```python
from build123d import *
from OCP.BRepFilletAPI import BRepFilletAPI_MakeChamfer

# Parameters (mm, degrees)
BOSS_EXTRU_1_DEPTH      = 200
BOSS_EXTRU_2_DEPTH      = 50
BOSS_EXTRU_2_DEPTH_BACK = 90
ESQUISSE3_W             = 40
ESQUISSE3_H             = 110
BOSS_EXTRU_3_DEPTH      = 150
CHANFREIN1_SIZE         = 10
CHANFREIN1_SIZE2        = 17.320508076
CHANFREIN2_SIZE         = 100
CHANFREIN2_SIZE2        = 46.630765816
CHANFREIN3_SIZE         = 10
CHANFREIN4_SIZE         = 30
BOSS_EXTRU_4_DEPTH      = 10
ENL_V_MAT_EXTRU_1_DEPTH = 130
ESQUISSE7_R             = 10
BOSS_EXTRU_5_DEPTH      = 30
CHANFREIN5_SIZE         = 27.474774195
CHANFREIN5_SIZE_2       = 10
ENL_V_MAT_EXTRU_2_DEPTH = 130
CHANFREIN6_SIZE         = 10
CHANFREIN6_SIZE_2       = 27.474774195
CHANFREIN6_SIZE_3       = 9.402654051


# Some blends are built 0.0001 mm under size
with BuildPart() as part:
    # Esquisse1 → Boss.-Extru.1 (new body)
    with BuildSketch(Plane.XY):
        Polygon((-42.05848897, 40), (-42.05848897, 0), (-37.05848897, 0), (-37.05848897, 5), (-37.05848897, 39.208077798), (-29.772778292, 61.631189606), (-11.372189368, 75), (11.372189368, 75), (29.772778292, 61.631189606), (37.05848897, 39.208077798), (37.05848897, 5), (37.05848897, 0), (42.05848897, 0), (42.05848897, 40), (34.026032334, 64.72135955), (12.996787849, 80), (-12.996787849, 80), (-34.026032334, 64.72135955), align=None)
    extrude(amount=BOSS_EXTRU_1_DEPTH)

    # Esquisse3 → Boss.-Extru.2 (add, two sides: drawn at the far end of the back side and taken through both)
    with BuildSketch(Plane(origin=(42.05848897, 0, 0), x_dir=(0, 0, -1), z_dir=(1, 0, 0)).offset(-BOSS_EXTRU_2_DEPTH_BACK)):
        with Locations((20, 45)):
            Rectangle(ESQUISSE3_W, ESQUISSE3_H)
    extrude(amount=BOSS_EXTRU_2_DEPTH + BOSS_EXTRU_2_DEPTH_BACK)

    # Esquisse4 → Boss.-Extru.3 (add)
    with BuildSketch(Plane.XY):
        Polygon((42.05848897, 40), (42.05848897, 15), (82.05848897, 15), (82.05848897, 65), (33.642516656, 65), (34.026032334, 64.72135955), align=None)
    extrude(amount=BOSS_EXTRU_3_DEPTH)

    # Chanfrein1: one chamfer whose edges measure the first distance from different faces: ONE call of the kernel's chamfer builder (chamfer() names one face for all edges)
    chanfrein1_edges_1 = [part.edges().sort_by_distance(p)[0] for p in [
        (92.05848897, -10, -20),
    ]]
    chanfrein1_side_1 = [part.faces().sort_by_distance(p)[0] for p in [
        (22.05848897, -10, -20),
    ]]
    chanfrein1_edges_2 = [part.edges().sort_by_distance(p)[0] for p in [
        (92.05848897, 100, -20),
    ]]
    chanfrein1_side_2 = [part.faces().sort_by_distance(p)[0] for p in [
        (22.05848897, 100, -20),
    ]]
    chanfrein1 = BRepFilletAPI_MakeChamfer(part.part.solid().wrapped)
    for e in chanfrein1_edges_1:
        chanfrein1.Add(CHANFREIN1_SIZE, CHANFREIN1_SIZE2, e.wrapped, chanfrein1_side_1[0].wrapped)  # the first distance lies on this face
    for e in chanfrein1_edges_2:
        chanfrein1.Add(CHANFREIN1_SIZE, CHANFREIN1_SIZE2, e.wrapped, chanfrein1_side_2[0].wrapped)  # the first distance lies on this face
    add(Compound.cast(chanfrein1.Shape()), mode=Mode.REPLACE)

    # Chanfrein2
    chanfrein2_edges = [part.edges().sort_by_distance(p)[0] for p in [
        (82.05848897, 40, 150),
    ]]
    chanfrein2_side = [part.faces().sort_by_distance(p)[0] for p in [
        (82.05848897, 40, 75),
    ]]
    chamfer(chanfrein2_edges, length=CHANFREIN2_SIZE, length2=CHANFREIN2_SIZE2, reference=chanfrein2_side[0])

    # Chanfrein3
    # the kernel refuses this chamfer: 10 mm, written as the material it takes off along each edge
    with BuildSketch(Plane(origin=(92.926890911, 15, 26.692636822), x_dir=(0.02491972708357348, 0.9996219169112968, 0.011620259578202877), z_dir=(-0.4226182617407005, 0, 0.9063077870366495))) as chanfrein3_piece_1_section:
        Polygon((CHANFREIN3_SIZE * 0.999621916911, CHANFREIN3_SIZE * 0.0274958766106), (-CHANFREIN3_SIZE * 0.0274958766106, CHANFREIN3_SIZE * 0.999621916911), (0, 0), align=None)
    chanfrein3_piece_1 = extrude(amount=146.081723085, mode=Mode.PRIVATE)
    chanfrein3_piece_1 = split(chanfrein3_piece_1, bisect_by=Plane(origin=(42.05848897, 18.333333333, 85.0027998), z_dir=(1, 0, 0)), keep=Keep.TOP, mode=Mode.PRIVATE)
    add(chanfrein3_piece_1, mode=Mode.SUBTRACT)
    with BuildSketch(Plane(origin=(82.05848897, 15, 0), x_dir=(0.027495876610586334, 0.9996219169112968, 0), z_dir=(0, 0, 1)), Plane(origin=(82.05848897, 65, 0), x_dir=(-0.9996219169112968, 0.027495876610586317, 0), z_dir=(0, 0, 1))) as chanfrein3_piece_2:
        Polygon((CHANFREIN3_SIZE * 0.999621916911, CHANFREIN3_SIZE * 0.0274958766106), (-CHANFREIN3_SIZE * 0.0274958766106, CHANFREIN3_SIZE * 0.999621916911), (0, 0), align=None)
    extrude(amount=75.71682988, mode=Mode.SUBTRACT)
    with BuildSketch(Plane(origin=(61.144553034, 65, 150), x_dir=(0, 0.027495876610586282, -0.9996219169112968), z_dir=(-1, 0, 0))) as chanfrein3_piece_3_section:
        Polygon((CHANFREIN3_SIZE * 0.999621916911, CHANFREIN3_SIZE * 0.0274958766106), (-CHANFREIN3_SIZE * 0.0274958766106, CHANFREIN3_SIZE * 0.999621916911), (0, 0), align=None)
    chanfrein3_piece_3 = extrude(amount=53.218866257, mode=Mode.PRIVATE)
    chanfrein3_piece_3 = split(chanfrein3_piece_3, bisect_by=Plane(origin=(34.447587874, 63.423945004, 144.130905286), z_dir=(0.9510565162951539, 0.3090169943749468, 0)), keep=Keep.TOP, mode=Mode.PRIVATE)
    add(chanfrein3_piece_3, mode=Mode.SUBTRACT)
    with BuildSketch(Plane(origin=(61.144553034, 65, 150), x_dir=(0, 0.027495876610586282, -0.9996219169112968), z_dir=(-1, 0, 0))) as chanfrein3_piece_4_section:
        Polygon((CHANFREIN3_SIZE * 0.999621916911, CHANFREIN3_SIZE * 0.0274958766106), (-CHANFREIN3_SIZE * 0.0274958766106, CHANFREIN3_SIZE * 0.999621916911), (0, 0), align=None)
    chanfrein3_piece_4 = extrude(amount=53.218866257, mode=Mode.PRIVATE)
    chanfrein3_piece_4 = split(chanfrein3_piece_4, bisect_by=Plane(origin=(33.833825058, 64.86100631, 145.046222385), z_dir=(0.5877852522924745, 0.8090169943749465, 0)), keep=Keep.TOP, mode=Mode.PRIVATE)
    add(chanfrein3_piece_4, mode=Mode.SUBTRACT)
    with BuildSketch(Plane(origin=(92.926890911, 65, 26.692636822), x_dir=(-0.9059651273892109, 0.027495876610586337, -0.4224584769229591), z_dir=(-0.4226182617407005, 0, 0.9063077870366495))) as chanfrein3_piece_5_section:
        Polygon((CHANFREIN3_SIZE * 0.999621916911, CHANFREIN3_SIZE * 0.0274958766106), (-CHANFREIN3_SIZE * 0.0274958766106, CHANFREIN3_SIZE * 0.999621916911), (0, 0), align=None)
    chanfrein3_piece_5 = extrude(amount=161.771451656, mode=Mode.PRIVATE)
    chanfrein3_piece_5 = split(chanfrein3_piece_5, bisect_by=Plane(origin=(37.356602315, 54.470919151, 89.132837903), z_dir=(0.9510565162951539, 0.3090169943749468, 0)), keep=Keep.TOP, mode=Mode.PRIVATE)
    add(chanfrein3_piece_5, mode=Mode.SUBTRACT)
    with BuildSketch(Plane(origin=(92.926890911, 65, 26.692636822), x_dir=(-0.9059651273892109, 0.027495876610586337, -0.4224584769229591), z_dir=(-0.4226182617407005, 0, 0.9063077870366495))) as chanfrein3_piece_6_section:
        Polygon((CHANFREIN3_SIZE * 0.999621916911, CHANFREIN3_SIZE * 0.0274958766106), (-CHANFREIN3_SIZE * 0.0274958766106, CHANFREIN3_SIZE * 0.999621916911), (0, 0), align=None)
    chanfrein3_piece_6 = extrude(amount=161.771451656, mode=Mode.PRIVATE)
    chanfrein3_piece_6 = split(chanfrein3_piece_6, bisect_by=Plane(origin=(33.834404205, 64.860585536, 139.950840197), z_dir=(0.5877852522924745, 0.8090169943749465, 0)), keep=Keep.TOP, mode=Mode.PRIVATE)
    add(chanfrein3_piece_6, mode=Mode.SUBTRACT)

    # Chanfrein4
    chanfrein4_edges = [part.edges().sort_by_distance(p)[0] for p in [
        (-39.55848897, 0, 200),
        (39.55848897, 0, 200),
    ]]
    chamfer(chanfrein4_edges, length=CHANFREIN4_SIZE)

    # Esquisse6 → Boss.-Extru.4 (add)
    with BuildSketch(Plane.XY):
        Polygon((-47.94151103, -10), (82.05848897, -10), (92.05848897, 7.320508076), (92.05848897, 82.679491924), (82.05848897, 100), (-47.94151103, 100), align=None)
    extrude(amount=BOSS_EXTRU_4_DEPTH)

    # Esquisse5 → Enlèv. mat.-Extru.1 (cut)
    with BuildSketch(Plane(origin=(0, 100, 0), x_dir=(1, 0, 0), z_dir=(0, 1, 0))):
        Polygon((77.05848897, -10), (77.05848897, 40), (-47.94151103, 40), (-47.94151103, -10), (33.642516656, -10), (67.05848897, -10), align=None)
        Polygon((67.05848897, -43.145928791), (67.05848897, -10), (33.642516656, -10), (33.642516656, -101.029300724), (42.077832628, -96.717119194), align=None)
    extrude(amount=-ENL_V_MAT_EXTRU_1_DEPTH, mode=Mode.SUBTRACT)

    # Esquisse7 → Boss.-Extru.5 (add)
    with BuildSketch(Plane.ZY.offset(-77.05848897)):
        with Locations(Location((-15, 80, 0), (0, 0, 270))):
            Circle(ESQUISSE7_R)
    extrude(amount=BOSS_EXTRU_5_DEPTH)

    # Chanfrein5
    chanfrein5_edges_1 = [part.edges().sort_by_distance(p)[0] for p in [
        (79.55848897, 22.5, 10),
    ]]
    chanfrein5_side_1 = [part.faces().sort_by_distance(p)[0] for p in [
        (79.55848897, 22.5, 10.2),
    ]]
    chanfrein5_edges_2 = [part.edges().sort_by_distance(p)[0] for p in [
        (82.05848897, 40, 10),
    ]]
    chanfrein5_side_2 = [part.faces().sort_by_distance(p)[0] for p in [
        (82.05848897, 40, 10.2),
    ]]
    chanfrein5_edges_3 = [part.edges().sort_by_distance(p)[0] for p in [
        (79.55848897, 57.5, 10),
    ]]
    chanfrein5_side_3 = [part.faces().sort_by_distance(p)[0] for p in [
        (79.55848897, 57.5, 10.2),
    ]]
    chanfrein5_edges_4 = [part.edges().sort_by_distance(p)[0] for p in [
        (67.05848897, 40, 10),
    ]]
    chanfrein5_side_4 = [part.faces().sort_by_distance(p)[0] for p in [
        (67.25848897, 40, 10),
    ]]
    chanfrein5 = BRepFilletAPI_MakeChamfer(part.part.solid().wrapped)
    for e in chanfrein5_edges_1:
        chanfrein5.Add(CHANFREIN5_SIZE - 0.0001, CHANFREIN5_SIZE_2 - 0.0001, e.wrapped, chanfrein5_side_1[0].wrapped)
    for e in chanfrein5_edges_2:
        chanfrein5.Add(CHANFREIN5_SIZE - 0.0001, CHANFREIN5_SIZE_2 - 0.0001, e.wrapped, chanfrein5_side_2[0].wrapped)
    for e in chanfrein5_edges_3:
        chanfrein5.Add(CHANFREIN5_SIZE - 0.0001, CHANFREIN5_SIZE_2 - 0.0001, e.wrapped, chanfrein5_side_3[0].wrapped)
    for e in chanfrein5_edges_4:
        chanfrein5.Add(CHANFREIN5_SIZE_2 - 0.0001, CHANFREIN5_SIZE - 0.0001, e.wrapped, chanfrein5_side_4[0].wrapped)
    add(Compound.cast(chanfrein5.Shape()), mode=Mode.REPLACE)  # a hair under: the kernel refuses the full size

    # Esquisse8 → Enlèv. mat.-Extru.2 (cut)
    with BuildSketch(Plane(origin=(0, 0, 0), x_dir=(1, 0, 0), z_dir=(0, 1, 0))):
        Polygon((-23.511410092, -10), (-23.511410092, -78.891987617), (-42.05848897, -124.008670609), (-42.05848897, -10), align=None)
    extrude(amount=ENL_V_MAT_EXTRU_2_DEPTH, mode=Mode.SUBTRACT)

    # Chanfrein6
    # the kernel refuses this chamfer: 27.474774195, 10, 9.402654051 mm, written as the material it takes off along each edge
    with BuildSketch(Plane(origin=(-23.511410092, -5.094574606, 10), x_dir=(0.9950833631817486, 0, -0.09904090225205081), z_dir=(0, 1, 0))) as chanfrein6_piece_1:
        Polygon((CHANFREIN6_SIZE * 0.995083363182, -CHANFREIN6_SIZE * 0.0990409022521), (-CHANFREIN6_SIZE_2 * 0.0990409022504, -CHANFREIN6_SIZE_2 * 0.995083363165), (0, 0), align=None)
    extrude(amount=148.730168875, mode=Mode.SUBTRACT)
    with BuildSketch(Plane(origin=(33.642516656, 136.274914494, 10), x_dir=(0.01318405819864584, 0, 0.9999130865277315), z_dir=(0, -1, 0))) as chanfrein6_piece_2:
        Polygon((CHANFREIN6_SIZE_2 * 0.999913086511, CHANFREIN6_SIZE_2 * 0.0131840581984), (-CHANFREIN6_SIZE * 0.0131840581986, CHANFREIN6_SIZE * 0.999913086528), (0, 0), align=None)
    extrude(amount=157.828469437, mode=Mode.SUBTRACT)
    with BuildSketch(Plane(origin=(-26.404734257, 0, 131.72579712), x_dir=(-0.04508122292734055, 0.9950833631817486, -0.08818607406090614), z_dir=(0.8904005522534487, -1.452228809103749e-15, -0.455177829586145))) as chanfrein6_piece_3:
        Polygon((CHANFREIN6_SIZE * 0.995083363182, CHANFREIN6_SIZE * 0.0990409022521), (-CHANFREIN6_SIZE_2 * 0.0990409022504, CHANFREIN6_SIZE_2 * 0.995083363165), (0, 0), align=None)
    extrude(amount=148.165279233, mode=Mode.SUBTRACT)
    # the kernel refuses this chamfer: 27.474774195, 10, 9.402654051 mm, written as the material it takes off along each edge
    with BuildSketch(Plane(origin=(33.642516656, 49.72135955, 12.11533794), x_dir=(-0.34404612147903313, 0.9389527497671193, 0), z_dir=(0, 0, 1))) as chanfrein6_2_piece_1_section:
        Polygon((CHANFREIN6_SIZE * 0.999313229545, -CHANFREIN6_SIZE * 0.0370549491456), (CHANFREIN6_SIZE_3 * 0.938952749733, -CHANFREIN6_SIZE_3 * 0.344046121466), (0, 0), align=None)
    chanfrein6_2_piece_1 = extrude(amount=114.273399039, mode=Mode.PRIVATE)
    chanfrein6_2_piece_1 = split(chanfrein6_2_piece_1, bisect_by=Plane(origin=(50.743372859, 55.917594233, 92.287245712), z_dir=(-0.455177829586145, 0, -0.8904005522534487)), keep=Keep.TOP, mode=Mode.PRIVATE)
    add(chanfrein6_2_piece_1, mode=Mode.SUBTRACT)


solid = part.part
```
Source: CAD feature listing. Evaluate the final solid. Frame: model axes, mm. A direction names the side the tool comes from. Give positions to 0.01 mm unless a question says otherwise; leave off trailing zeros. Order: outer loops, then holes, each group sorted by start corner. A loop starts at its lowest first (then second) coordinate and runs counter-clockwise, first axis right, second up. Notation, with made-up numbers: (39, 80) -> (89, 80) arc R20 cw to (89, 97) -> close; hole circle Ø6 at (-23, 33.5). An arc over 180 degrees is marked (long way). Use a Markdown table: item, result.
Q1. Section D-D (x = 9). Return the cut outline in (y, z).
A:
| item | result |
|---|---|
| outline | (75, 10) -> (80, 10) -> (80, 200) -> (75, 200) -> close |
Q2. First-contact query: P1, Ø8, axis at x = 58.5, y = 87, coming from the -Z side; P2, Ø11.5, axis at x = 52, z = 66.5, coming from the +Y side; P3, Ø10, axis at y = 41, z = 46, coming from the +X side; P4, Ø12, axis at x = 59.5, z = 34, coming from the +Y side. Flat tips, straight axial feed; report the tip coordinate or a pass-through.
A:
| item | result |
|---|---|
| P1 | z = -24.54 |
| P2 | y = 65 |
| P3 | x = 82.06 |
| P4 | through |
Q3. Access query for faces 1 (the face through (5, 76, 10)), 2 (the face through (62, 90, -15)), 3 (the face through (-37.058, 19, 155)), 4 (the face through (82.058, 40, 44)), 5 (the face through (86.99, -1.46, -15.35)). Directions: +Z, -Z, +X, -X, +Y, -Y. A direction counts if a zero-diameter tool reaches every point of the face in a straight line with its end or side. Return the directions, or none.
A:
| item | result |
|---|---|
| face 1 | -Z, -X, +Y, -Y |
| face 2 | -X |
| face 3 | +Z, -Z, -Y |
| face 4 | +Z, +X, +Y, -Y |
| face 5 | +Z, -Z, +X, -Y |
Q4. Material intervals for line 1 (X direction, y = 18.5, z = 161); line 2 (X direction, y = 73.5, z = 17); line 3 (X direction, y = 77, z = -9), sorted ascending. Write a range as [from, to].
A:
| item | result |
|---|---|
| line 1 | [-42.06, -37.06], [37.06, 42.06] |
| line 2 | [-16.06, -13.44], [13.44, 21.94] |
| line 3 | [47.06, 92.06] |
Q5. Section A-A (z = 88.5). Return the cut outline in (x, y).
A:
| item | result |
|---|---|
| outline | (-27.46, 63.31) -> (-11.37, 75) -> (11.37, 75) -> (29.77, 61.63) -> (30.55, 59.23) -> (33.64, 59.12) -> (33.64, 65) -> (13, 80) -> (-13, 80) -> (-27.46, 69.49) -> close; (45.91, 15) -> (53.07, 15) -> (64.11, 25) -> (64.11, 55) -> (53.07, 65) -> (45.91, 65) -> close |
Q6. Section B-B (x = 50). Return the cut outline in (y, z), and give its area (3 significant figures).
A:
| item | result |
|---|---|
| outline | (15, 79.73) -> (65, 79.73) -> (65, 95.09) -> (55, 118.75) -> (25, 118.75) -> (15, 95.09) -> close; circle Ø20 at (80, -15) |
| area | 2,030 mm^2 |
Q7. Section C-C (z = 3). Return the cut outline in (x, y).
A:
| item | result |
|---|---|
| outline | (77.06, -10) -> (82.06, -10) -> (92.06, 7.32) -> (92.06, 82.68) -> (82.06, 100) -> (77.06, 100) -> close |
Q8. Pull-direction query (X, two-part tool) for faces 6 (the face through (33.643, 62, 69)), 7 (the face through (-23.511, 69, 58)), 8 (the face through (83.42, 62.38, 20.49)); classes: +X half, -X half, draft (parallel to the pull), parting line (faces both ways), or undercut.
A:
| item | result |
|---|---|
| face 6 | undercut |
| face 7 | -X half |
| face 8 | +X half |
